Here's how the part is built. I have some questions about the finished solid (model axes, mm). Round coordinates to 2 decimals unless told otherwise and drop trailing zeros. Loops run counter-clockwise (first coordinate to the right, second up) from the corner with the lowest first, then second, coordinate; pieces in that order, holes last. Notation, with made-up numbers: (5.5, 10.5) - (40.5, 10.5) arc R20 cw to (40.5, 45.5) - close; hole circle Ø8 at (-23.5, 18). An arc over 180 degrees is marked (long way). Return JSON: item names as keys, results as strings. Group by question number.
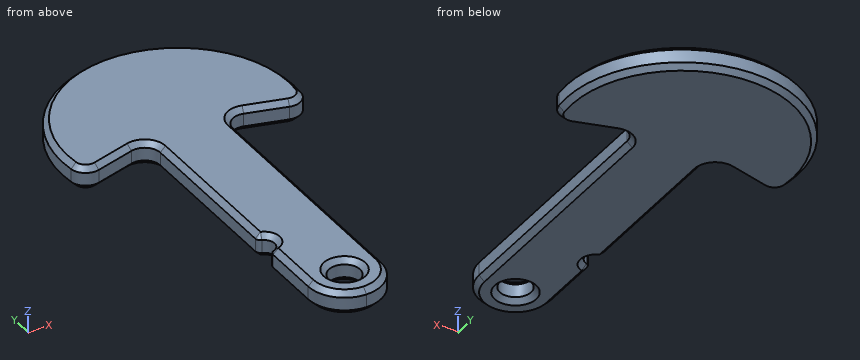
```python
from build123d import *

# Parameters (mm, degrees)
F0_R     = 1.5
F1_DEPTH = 2.25
F2_R     = 1.5
F3_SIZE  = 0.49999


# Not quite as in the source:
# - a fillet or chamfer is up to 0.001 mm smaller than in the source, because OpenCascade refuses the exact size


with BuildPart() as f1:
    # F0 (on Top) → F1 (new body)
    with BuildSketch(Plane.XY):
        with BuildLine():
            Line((3.5, -0.9777600189), (10.7388314076, -3))
            ThreePointArc((10.7388314076, -3), (0, 11.15), (-10.7388314076, -3))
            Line((-10.7388314076, -3), (-3.5, -0.9777600189))
            Line((-3.5, -0.9777600189), (-3.5, -18.0857864376))
            ThreePointArc((-3.5, -18.0857864376), (-3.4082482905, -18.3744615722), (-3.1666666667, -18.5571909584))
            ThreePointArc((-3.1666666667, -18.5571909584), (-2.5, -19.5), (-3.1666666667, -20.4428090416))
            ThreePointArc((-3.1666666667, -20.4428090416), (-3.4082482905, -20.6255384278), (-3.5, -20.9142135624))
            Line((-3.5, -20.9142135624), (-3.5, -26.5))
            ThreePointArc((-3.5, -26.5), (-2.4748737342, -28.9748737342), (0, -30))
            ThreePointArc((0, -30), (2.4748737342, -28.9748737342), (3.5, -26.5))
            Line((3.5, -26.5), (3.5, -0.9777600189))
        make_face()
        with Locations((0, -26.5)):
            Circle(F0_R, mode=Mode.SUBTRACT)
    extrude(amount=F1_DEPTH)

    # F2
    f2_edges = [f1.edges().sort_by_distance(p)[0] for p in [
        (10.738831, -3, 1.125),
        (-10.738831, -3, 1.125),
        (-3.5, -0.97776, 1.125),
        (3.5, -0.97776, 1.125),
    ]]
    fillet(f2_edges, radius=F2_R)

    # F3 (size 0.5 in the source; OpenCascade refuses exactly that, so slightly less here)
    f3_edges = [f1.edges().sort_by_distance(p)[0] for p in [
        (3.5, -14.727116, 2.25),
        (4.093187, -1.759372, 2.25),
        (0, -30, 2.25),
        (7.292383, -2.0372, 2.25),
        (-3.5, -23.707107, 2.25),
        (10.420577, -2.365727, 2.25),
        (-3.408248, -20.625538, 2.25),
        (0, 11.15, 2.25),
        (-2.5, -19.5, 2.25),
        (-10.420577, -2.365727, 2.25),
        (-3.408248, -18.374462, 2.25),
        (-7.292383, -2.0372, 2.25),
        (-3.5, -10.520009, 2.25),
        (-4.093187, -1.759372, 2.25),
        (-1.5, -26.5, 2.25),
        (3.5, -14.727116, 0),
        (4.093187, -1.759372, 0),
        (0, -30, 0),
        (7.292383, -2.0372, 0),
        (-3.5, -23.707107, 0),
        (10.420577, -2.365727, 0),
        (-3.408248, -20.625538, 0),
        (0, 11.15, 0),
        (-2.5, -19.5, 0),
        (-10.420577, -2.365727, 0),
        (-3.408248, -18.374462, 0),
        (-7.292383, -2.0372, 0),
        (-3.5, -10.520009, 0),
        (-4.093187, -1.759372, 0),
        (-1.5, -26.5, 0),
    ]]
    chamfer(f3_edges, length=F3_SIZE)


solid = f1.part
```
Q1. Imagine slicing it at A-A, the plane z = 0.95. List the corners of the cut face in (x, y) for me, and give its area (3 significant figures).
Q2. Please list where these lines run through material, in increasing order: line 1 (X direction, y = -3, z = 1.6); line 2 (Y direction, x = -9.75, z = 1.05); line 3 (Y direction, x = -0.75, z = 0.9).
Q3. Will these pins go through, and if not, where does the flat tip stop? pin 1 Ø0.6 at (y, z) = (-18, 1) entering from +X; pin 2 Ø1 at (y, z) = (2, 0.5) entering from -X; pin 3 Ø1 at (y, z) = (-11.5, 1.5) entering from -X.
Q4. Imagine slicing it at B-B, the plane y = -22.5. List the corners of the cut face in (x, z) for me.
Output values:
{
 "1": {"outline": "(-11.07, -1.29) arc R1.5 ccw to (-9.18, -2.56) - (-5.4, -1.51) arc R1.5 cw to (-3.5, -2.95) - (-3.5, -18.09) arc R0.5 ccw to (-3.17, -18.56) arc R1 cw to (-3.17, -20.44) arc R0.5 ccw to (-3.5, -20.91) - (-3.5, -26.5) arc R3.5 ccw to (3.5, -26.5) - (3.5, -2.95) arc R1.5 cw to (5.4, -1.51) - (9.18, -2.56) arc R1.5 ccw to (11.07, -1.29) arc R11.15 ccw (long way) to start; hole circle Ø3 at (0, -26.5)", "area": "422 mm^2"},
 "2": {"line 1": "x = -3.5 to 3.5", "line 2": "y = -2.61 to 5.41", "line 3": "y = -29.92 to -27.8, -25.2 to 11.12"},
 "3": {"pin 1": "stops at x = 3.5", "pin 2": "stops at x = -11.05", "pin 3": "stops at x = -3.5"},
 "4": {"outline": "(-3.5, 0.5) - (-3, 0) - (3, 0) - (3.5, 0.5) - (3.5, 1.75) - (3, 2.25) - (-3, 2.25) - (-3.5, 1.75) - close"}
}
